Answer from the drawing. Dimensions are ordinates in mm from the lowest x, y and z of the part. A direction names the side the tool comes from. Give positions to 0.01 mm unless a question says otherwise; leave off trailing zeros. Loops run counter-clockwise (first coordinate to the right, second up) from the corner with the lowest first, then second, coordinate; pieces in that order, holes last. Notation, with made-up numbers: (31, -39.75) - (46, -39.75) arc R19 cw to (46, -30.75) - close; hole circle Ø10 at (89.5, 1). An arc over 180 degrees is marked (long way). Answer as CSV lines item,"result". Start each with the question number.
1) A cutting plane is placed at A-A (y = 16). Determine the outline of the cut face in (x, z), and give its area (3 significant figures).
2) For a pull along Y with two mould halves and no side action, classify the marked faces 1, 2 and 3 as pulls with the +Y half, pulls with the -Y half, needs draft (parallel to the pull), parting line crosses it, or undercut.
3) A cutting plane is placed at C-C (z = 5.5). Determine the outline of the cut face in (x, y).
4) Find the intervals of material crossed by line 1 along Y through (x, z) = (18, 5.25); line 2 along X through (y, z) = (66, 9.25); line 3 along X through (y, z) = (62.5, 6.5), in increasing order.
5) A cutting plane is placed at B-B (x = 118). Determine the outline of the cut face in (y, z).
6) For the marked faces 4, 5, 6, 7 and 8, determine the directions among +Z, -Z, +X, -X, +Y, -Y from which every point of the face is accessible in a straight line to the end or side of a thin tool.
7) Flat-ended cylindrical pins translate along their axes: pin 1 (16 mm diameter, centred on x = 99, y = 27, fed in from +Z); pin 2 (13.5 mm diameter, centred on x = 18, y = 16, fed in from +Z); pin 3 (7.5 mm diameter, centred on x = 74, y = 33.5, fed in from -Z). Find the tip coordinate at first contact, or state that the pin passes through.
8) A cutting plane is placed at D-D (y = 35.5). Determine the outline of the cut face in (x, z).
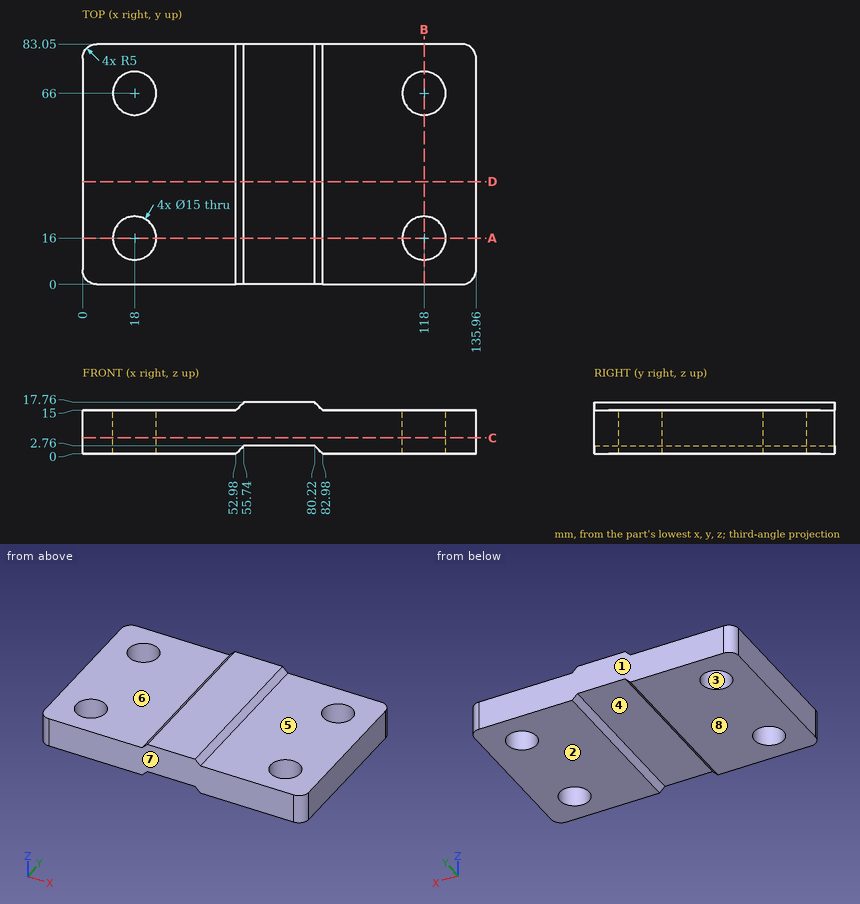
Ans:
1,outline,"(0, 0) - (10.5, 0) - (10.5, 15) - (0, 15) - close; (25.5, 0) - (52.98, 0) - (55.74, 2.76) - (80.22, 2.76) - (82.98, 0) - (110.5, 0) - (110.5, 15) - (82.98, 15) - (80.22, 17.76) - (55.74, 17.76) - (52.98, 15) - (25.5, 15) - close; (125.5, 0) - (135.96, 0) - (135.96, 15) - (125.5, 15) - close"
1,area,"1,590 mm2"
2,face 1,"pulls with the +Y half"
2,face 2,"needs draft"
2,face 3,"undercut"
3,outline,"(0, 5) arc R5 ccw to (5, 0) - (130.96, 0) arc R5 ccw to (135.96, 5) - (135.96, 78.05) arc R5 ccw to (130.96, 83.05) - (5, 83.05) arc R5 ccw to (0, 78.05) - close; hole circle Ø15 at (18, 16); hole circle Ø15 at (18, 66); hole circle Ø15 at (118, 16); hole circle Ø15 at (118, 66)"
4,line 1,"0 to 8.5, 23.5 to 58.5, 73.5 to 83.05"
4,line 2,"0 to 10.5, 25.5 to 110.5, 125.5 to 135.96"
4,line 3,"0 to 11.37, 24.63 to 111.37, 124.63 to 135.96"
5,outline,"(0, 0) - (8.5, 0) - (8.5, 15) - (0, 15) - close; (23.5, 0) - (58.5, 0) - (58.5, 15) - (23.5, 15) - close; (73.5, 0) - (83.05, 0) - (83.05, 15) - (73.5, 15) - close"
6,face 4,"-Z, +Y, -Y"
6,face 5,"+Z, +X, +Y, -Y"
6,face 6,"+Z, -X, +Y, -Y"
6,face 7,"+Z, -Z, +X, -X, -Y"
6,face 8,"-Z, +X, -X, +Y, -Y"
7,pin 1,"z = 15"
7,pin 2,"through"
7,pin 3,"z = 2.76"
8,outline,"(0, 0) - (52.98, 0) - (55.74, 2.76) - (80.22, 2.76) - (82.98, 0) - (135.96, 0) - (135.96, 15) - (82.98, 15) - (80.22, 17.76) - (55.74, 17.76) - (52.98, 15) - (0, 15) - close"
